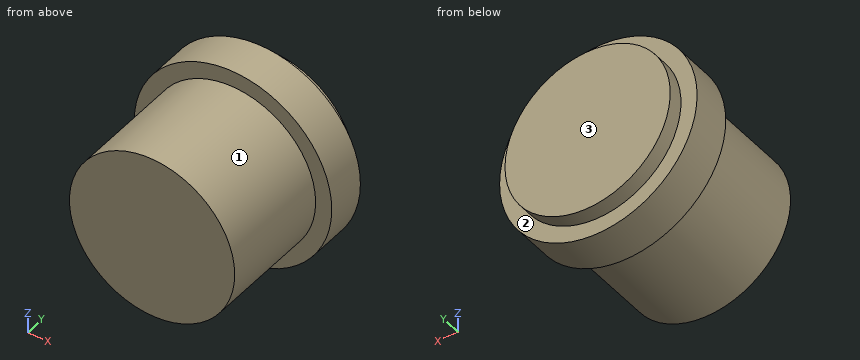
Autodesk Fusion 360 part; units mm, degrees
sketch "Sketch1" plane through (0, 0, 0) normal (0, 1, 0) x (1, 0, 0)
  circle A0 centre (0, 0) radius 4.1
  dimension "d2" = 8.2
extrude "Extrude1" add sketch "Sketch1" along normal blind 8.4
sketch "Sketch2" plane through (0, 8.4, 0) normal (0, 1, 0) x (-1, 0, 0)
  circle A0 centre (0, 0) radius 4.1
  circle A1 centre (0, 0) radius 4.9
  dimension "d5" = 9.8
extrude "Extrude2" add sketch "Sketch2" against normal blind 2 from surface at -0.75
equation "ActuatorDepth = 0.75 mm"
The listing builds one solid part. Answer for the finished solid, in the listing's coordinates (mm). Face numbers are marked on the shaded views. A direction names the side the tool comes from. Coordinates: 2 decimals unless noted, no trailing zeros. Loops run counter-clockwise (first coordinate to the right, second up) from the corner with the lowest first, then second, coordinate; pieces in that order, holes last. Notation, with made-up numbers: M 39,-28.75 L 68,-28.75 A29 cw 68,6.25 Z; hole C 18,-40 d6. An arc over 180 degrees is marked long. Answer in a Markdown table with one row per item.
1) Find section D-D (y = 6). Determine the outline of the cut face in (x, z).
Answers below:
| item | result |
|---|---|
| outline | C 0,0 d9.8 |
2) Find section B-B (z = 0). Determine the outline of the cut face in (x, y), then the cut area to 3 significant figures.
Answers below:
| item | result |
|---|---|
| outline | M -4.9,5.65 L -4.1,5.65 L -4.1,0 L 4.1,0 L 4.1,5.65 L 4.9,5.65 L 4.9,7.65 L 4.1,7.65 L 4.1,8.4 L -4.1,8.4 L -4.1,7.65 L -4.9,7.65 Z |
| area | 72.1 mm^2 |
3) Find the intervals of material crossed by probe 1 along X at (y, z) = (4.75, 0); probe 2 along Z at (x, y) = (-1.5, 3.5); probe 3 along X at (y, z) = (5.5, -3.25), in increasing order.
Answers below:
| item | result |
|---|---|
| probe 1 | -4.1 to 4.1 |
| probe 2 | -3.82 to 3.82 |
| probe 3 | -2.5 to 2.5 |
4) Given pin 1 (4 mm diameter, centred on y = 1.5, z = -0.5, fed in from -X); pin 2 (2 mm diameter, centred on x = 3.5, z = -2, fed in from -Y); pin 3 (4 mm diameter, centred on y = 3, z = -1, fed in from +X); pin 4 (2 mm diameter, centred on y = 2.5, z = -2.5, fed in from -X), each flat-ended and moving along its own axis, determine where each tip first touches the part or whether it passes through.
Answers below:
| item | result |
|---|---|
| pin 1 | x = -4.1 |
| pin 2 | y = 0 |
| pin 3 | x = 4.1 |
| pin 4 | x = -3.82 |
5) Find section C-C (y = 3). Determine the outline of the cut face in (x, z), then the cut area to 3 significant figures.
Answers below:
| item | result |
|---|---|
| outline | C 0,0 d8.2 |
| area | 52.8 mm^2 |
6) Find section A-A (x = 0). Determine the outline of the cut face in (y, z), then the cut area to 3 significant figures.
Answers below:
| item | result |
|---|---|
| outline | M 0,-4.1 L 5.65,-4.1 L 5.65,-4.9 L 7.65,-4.9 L 7.65,-4.1 L 8.4,-4.1 L 8.4,4.1 L 7.65,4.1 L 7.65,4.9 L 5.65,4.9 L 5.65,4.1 L 0,4.1 Z |
| area | 72.1 mm^2 |
7) Which of the six approach directions +Z, -Z, +X, -X, +Y, -Y give full straight-line access (tool end or side, diameter ignored) to the marked faces 1, 2 and 3?
Answers below:
| item | result |
|---|---|
| face 1 | -Y |
| face 2 | +Y |
| face 3 | +Z, -Z, +X, -X, +Y |
